Source: CAD feature listing. Evaluate the final solid. Frame: model axes, mm. A direction names the side the tool comes from. Give positions to 0.01 mm unless a question says otherwise; leave off trailing zeros. Write each loop counter-clockwise with the first axis right and the second up, starting at its lowest first coordinate (ties: lowest second). Pieces come first, ordered by that corner, then holes.
Autodesk Inventor part; units mm, degrees
ref_plane "Work Plane1" through (34.2931, 25.9114, -33.2342) normal (0, 1, 0) x (-1, 0, 0)
ref_plane "작업 평면2" through (3.5431, 25.6014, -33.2342) normal (0, 0, 1) x (1, 0, 0)
ref_plane "YZ Plane" through (0, 0, 0) normal (1, 0, 0) x (0, 1, 0)
ref_plane "Work Plane1" through (34.2931, 25.9114, -33.2342) normal (0, 1, 0) x (-1, 0, 0)
sketch "Sketch2" plane through (34.2931, 25.9114, -33.2342) normal (0, 1, 0) x (-1, 0, 0)
  circle A0 centre (9.75, 7.1) radius 0.7835
  circle A1 centre (16.85, 0) radius 0.7835
  circle A2 centre (9.75, -7.1) radius 0.7835
  circle A3 centre (2.65, 0) radius 0.7835
  circle A4 centre (4.7295, -5.0205) radius 0.7835
  circle A5 centre (14.7705, -5.0205) radius 0.7835
  circle A6 centre (14.7705, 5.0205) radius 0.7835
  circle A7 centre (4.7295, 5.0205) radius 0.7835
  circle A8 centre (9.75, 0) radius 3.8
  circle A9 centre (9.75, 0) radius 9.75
  circle A10 centre (9.75, 0) radius 2.75
  line L0 (30.75, -10.5) -> (30.75, 10.5)
  line L1 (30.75, -10.5) -> (25.75, -10.5)
  line L2 (30.75, 10.5) -> (25.75, 10.5)
  line L3 (25.75, -10.5) -> (9.2998, -9.7396)
  line L4 (25.75, 10.5) -> (9.2998, 9.7396)
  circle A11 centre (16.85, 0) radius 1.05
  circle A12 centre (9.75, 7.1) radius 1.05
  circle A13 centre (2.65, 0) radius 1.05
  circle A14 centre (9.75, -7.1) radius 1.05
  point P0 (34.2931, 33.2342)
  point P1 (30.75, 0)
  dimension "d2" = 5.5
  dimension "d4" = 21
  dimension "d5" = 5
  dimension "d6" = 21
  dimension "d37" = 2.1
extrude "Plate2" add sketch "Sketch2" along normal blind 1.5 contours A4 | A5 | A6 | A7 | A8 | A9 | A9 L4 L2 L0 L1 L3
sketch "Sketch3" plane through (5.0431, 27.4114, -43.7342) normal (-1, 0, 0) x (0, -1, 0)
  line L0 (0, 21) -> (0, 0)
  line L1 (0, 0) -> (55, 0)
  line L2 (55, 0) -> (55, 21)
  line L3 (55, 21) -> (0, 21)
edge flange "Flange1" height 55 angle 90 thickness 1.5 bend radius 0.31 thickness toward (-1, 0, 0) relief tear relief width 1.5 relief depth 0.75 edges at (3.5431, 25.9114, -33.2342) wall of the first edge with corners at (5.0431, 27.4114, -22.7342) (5.0431, 27.4114, -43.7342) (5.0431, -27.5886, -43.7342) (5.0431, -27.5886, -22.7342)
bend "Bend1"
corner "Corner1"
sketch "Sketch4" plane through (3.5431, -26.0886, -43.7342) normal (0, -1, 0) x (1, 0, 0)
  line L0 (0, 21) -> (0, 0)
  line L1 (0, 0) -> (35, 0)
  line L2 (35, 0) -> (35, 21)
  line L3 (35, 21) -> (0, 21)
edge flange "Flange2" height 35 angle 90 thickness 1.5 bend radius 0.31 thickness toward (0, -1, 0) relief tear relief width 1.5 relief depth 0.75 edges at (5.0431, -27.5886, -33.2342) wall of the first edge with corners at (3.5431, -26.0886, -22.7342) (3.5431, -26.0886, -43.7342) (38.5431, -26.0886, -43.7342) (38.5431, -26.0886, -22.7342)
bend "Bend2"
corner "Corner2"
sketch "Sketch5" plane through (38.5431, -27.5886, -43.7342) normal (0, -1, 0) x (1, 0, 0)
  circle A0 centre (-14, 10.5) radius 3.85
  point P0 (-38.5431, 43.7342)
extrude "Cut1" cut sketch "Sketch5" against normal blind 1.5
sketch "Sketch6" plane through (38.5431, -27.5886, -43.7342) normal (0, -1, 0) x (1, 0, 0)
  line L0 (-33.19, 0) -> (-33.19, 21)
  line L1 (-30, 21) -> (-33.19, 21)
  line L2 (-13.5498, 20.2396) -> (-30, 21)
  arc A0 (-13.5498, 0.7604) -> (-13.5498, 20.2396) centre (-14, 10.5) ccw
  line L3 (-30, 0) -> (-13.5498, 0.7604)
  line L4 (-33.19, 0) -> (-30, 0)
  line L5 (-90, -199.5) -> (-90, 50.5)
  line L6 (220, -199.5) -> (-90, -199.5)
  circle A1 centre (-14, 17.525) radius 0.7835
  circle A2 centre (-6.975, 10.5) radius 0.7835
  circle A3 centre (-14, 3.475) radius 0.7835
  circle A4 centre (-21.025, 10.5) radius 0.7835
  circle A5 centre (-6.975, 10.5) radius 1.05
  circle A6 centre (-14, 17.525) radius 1.05
  circle A7 centre (-21.025, 10.5) radius 1.05
  circle A8 centre (-14, 3.475) radius 1.05
  line L7 (-33.19, 21) -> (0, 21)
  line L8 (0, 21) -> (0, 0)
  line L9 (0, 0) -> (-33.19, 0)
  line L10 (220, -199.5) -> (220, 50.5)
  line L11 (220, 50.5) -> (-90, 50.5)
  point P0 (-38.5431, 43.7342)
  dimension "d38" = 2.1
extrude "Cut2" cut sketch "Sketch6" against normal blind 1.5 contours L3 A0 L2 L7 L8 L9 | A1 | A2 | A3 | A4 | A5 | A6 | A7 | A8
ref_plane "작업 평면2" through (3.5431, 25.6014, -33.2342) normal (0, 0, 1) x (1, 0, 0)
sketch "Sketch7" plane through (5.0431, 25.6014, -22.7342) normal (1, 0, 0) x (0, 0, -1)
  line L0 (0, -51.38) -> (21, -51.38)
  line L1 (21, 0) -> (21, -51.38)
  line L2 (21, 0) -> (0, 0)
  line L3 (0, 0) -> (0, -51.38)
  line L4 (10.5, 0) -> (10.5, -51.38) construction
  circle A0 centre (10.5, -25.69) radius 2
  circle A1 centre (10.5, -7.69) radius 2
  circle A2 centre (10.5, -43.69) radius 2
  point P0 (-22.7342, -25.6014)
  dimension "d32" = 18
  dimension "d33" = 18
  dimension "d34" = 4
extrude "Cut3" cut sketch "Sketch7" against normal blind 1.5 contours A0 | A1 | A2
equation "\"d28\" = Thickness"
equation "\"d30\" = Thickness"
equation "\"d35\" = Thickness"
equation "\"d7\" = Thickness"
equation "\"d8\" = BendReliefWidth"
equation "\"d9\" = BendReliefDepth"
equation "\"d10\" = MinimumRemnant"
equation "\"d11\" = TransitionRadius"
equation "\"d14\" = BendRadius"
equation "\"d15\" = CornerReliefSize"
equation "\"d16\" = GapSize"
equation "\"d17\" = JacobiRadiusSize"
equation "\"d18\" = BendReliefWidth"
equation "\"d19\" = BendReliefDepth"
equation "\"d20\" = MinimumRemnant"
equation "\"d21\" = TransitionRadius"
equation "\"d24\" = BendRadius"
equation "\"d25\" = CornerReliefSize"
equation "\"d26\" = GapSize"
equation "\"d27\" = JacobiRadiusSize"
equation "\"BendReliefWidth\" = Thickness"
equation "\"BendReliefDepth\" = 0.5 * Thickness"
equation "\"CornerReliefSize\" = 4 * Thickness"
equation "\"MinimumRemnant\" = 2 * Thickness"
equation "\"TransitionRadius\" = BendRadius"
equation "\"JacobiRadiusSize\" = BendRadius"
equation "\"GapSize\" = Thickness"
properties part number "ㄷ_frame_1" material "Aluminum 6061"
1. Section query B-B (x = 26.5). Return loops of the section in (y, z).
2. Line query: probe 1 along Y at (x, z) = (10.5, -29.5); probe 2 along X at (y, z) = (14.5, -42.25); probe 3 along Y at (x, z) = (21.5, -33.5). Output: solid intervals per line, ascending.
3. Section query C-C (y = -14). Return loops of the section in (x, z), plus the area to 3 significant figures.
4. Access query for faces 1 (the cylindrical face through (24.77, 26.65, -25.11)), 2 (the cylindrical face through (20.697, -26.849, -33.065)), 3 (the flat face through (20, 25.911, -33)). Directions: +Z, -Z, +X, -X, +Y, -Y. A direction counts if a zero-diameter tool reaches every point of the face in a straight line with its end or side. Return the directions, or none.
5. Section query A-A (x = 22.5). Return loops of the section in (y, z).
6. Pull-direction query (Y, two-part tool) for faces 4 (the flat face through (5.043, 0, -31)), 5 (the cylindrical face through (4.304, -0.001, -31.236)), 6 (the cylindrical face through (25.32, 26.65, -41.04)), 7 (the cylindrical face through (4.087, -27.072, -33.381)); classes: pulls with the +Y half, pulls with the -Y half, needs draft (parallel to the pull), parting line crosses it, or undercut.
7. Pin query (flat end, axial travel): P1, Ø6, axis at y = 20, z = -30.5, coming from the +X side; P2, Ø10.5, axis at x = 23.5, z = -31, coming from the -Y side; P3, Ø6, axis at x = 24.54, z = -33.23, coming from the -Y side. Return the tip coordinate at first contact, or that it passes through.
The answers:
1. outline: (-27.59, -42.79) - (-26.09, -42.79) - (-26.09, -36.55) - (-27.59, -36.55) - close; (-27.59, -29.92) - (-26.09, -29.92) - (-26.09, -23.68) - (-27.59, -23.68) - close; (25.91, -42.79) - (27.41, -42.79) - (27.41, -35.17) - (25.91, -35.17) - close; (25.91, -31.3) - (27.41, -31.3) - (27.41, -23.68) - (25.91, -23.68) - close
2. probe 1: y = -27.59 to -26.09, 25.91 to 27.41
2. probe 2: x = 3.54 to 5.04
2. probe 3: y = 25.91 to 27.41
3. outline: (3.54, -43.73) - (5.04, -43.73) - (5.04, -22.73) - (3.54, -22.73) - close
3. area: 31.5 mm2
4. face 1: +Y
4. face 2: -Y
4. face 3: +Z, -Z, +X
5. outline: (-27.59, -43.09) - (-26.09, -43.09) - (-26.09, -36.5) - (-27.59, -36.5) - close; (-27.59, -29.97) - (-26.09, -29.97) - (-26.09, -23.38) - (-27.59, -23.38) - close; (25.91, -43.09) - (27.41, -43.09) - (27.41, -35.07) - (25.91, -35.07) - close; (25.91, -31.39) - (27.41, -31.39) - (27.41, -23.38) - (25.91, -23.38) - close
6. face 4: undercut
6. face 5: undercut
6. face 6: needs draft
6. face 7: pulls with the -Y half
7. P1: stops at x = 5.04
7. P2: stops at y = -27.59
7. P3: stops at y = 25.91
